Read the model definition and answer for the solid it produces. Units are mm, in the model's axes. A direction names the side the tool comes from. Round coordinates to 2 decimals unless told otherwise and drop trailing zeros. Write each loop counter-clockwise with the first axis right and the second up, starting at its lowest first coordinate (ties: lowest second). Pieces come first, ordered by that corner, then holes. Notation, with made-up numbers: (69, 80.5) - (75, 80.5) arc R33 cw to (75, 116.5) - close; hole circle Ø10 at (57, 1). An arc over 180 degrees is marked (long way). Use one line per item in the form item = value. Start each with the question number.
1) The part is cut by section C-C, the plane x = 60. Give the vertices of the cut face in (y, z).
2) The part is cut by section D-D, the plane y = -129.5. Give the vertices of the cut face in (x, z), plus the area to 3 significant figures.
3) Each of these flat-tipped pins is pushed along its axis until it touches: pin 1 (11 mm diameter, centred on x = 110, y = -73.5, fed in from -Z); pin 2 (6 mm diameter, centred on x = 11.5, z = 70, fed in from +Y); pin 3 (16 mm diameter, centred on x = 58, z = 13, fed in from -Y); pin 4 (2 mm diameter, centred on x = 89.5, y = -65, fed in from +Z). Where does it stop, or does it pass through?
4) The part is cut by section A-A, the plane y = -50.5. Give the vertices of the cut face in (x, z).
5) Consider line 1 along Y through (x, z) = (73, 228.5); line 2 along Z through (x, y) = (13, -100); line 3 along Y through (x, z) = (16, 213). Determine where each line is inside the solid, lowest interval first. Write a range as from..to.
6) For a pull along Z with two mould halves and no side action, classify faces 1 (the face through (113, -74, 170)), 2 (the face through (60, -48, 270)), 3 (the face through (25, -138, 10)) as released by +Z, released by -Z, zero draft, split by the parting line, or undercut.
7) For faces 4 (the face through (35, -23, 10)), 5 (the face through (30, -15, 233)), 6 (the face through (40, -20, 232)), determine the directions among +Z, -Z, +X, -X, +Y, -Y from which every point of the face is accessible in a straight line to the end or side of a thin tool.
8) The part is cut by section B-B, the plane z = 72.5. Give the vertices of the cut face in (x, y), plus the area to 3 significant figures.
from build123d import *

# Parameters (mm, degrees)
SKETCH_1_W          = 120
SKETCH_1_H          = 150
EXTRUDE_1_DEPTH     = 20
SKETCH_2_W          = 120
SKETCH_2_H          = 10
EXTRUDE_3_DEPTH     = 250
SKETCH_3_W          = 50
SKETCH_3_H          = 45
CUT_EXTRUDE_1_DEPTH = 316.277655409
SKETCH_4_W          = 70
SKETCH_4_H          = 25
CUT_EXTRUDE_2_DEPTH = 316.277655409
SKETCH_5_W          = 20
SKETCH_5_H          = 20
CUT_EXTRUDE_3_DEPTH = 3
CUT_EXTRUDE_START   = -100
CUT_EXTRUDE_6_DEPTH = 20
SKETCH_7_W          = 20
SKETCH_7_H          = 75
EXTRUDE_4_DEPTH     = 50
SKETCH_8_W          = 60
SKETCH_8_H          = 75
EXTRUDE_5_DEPTH     = 10


with BuildPart() as part:
    # Эскиз1 → Бобышка-Вытянуть1 (new body)
    with BuildSketch(Plane.XY):
        with Locations((60, -75)):
            Rectangle(SKETCH_1_W, SKETCH_1_H)
    extrude(amount=EXTRUDE_1_DEPTH)

    # Эскиз2 → Бобышка-Вытянуть3 (add)
    with BuildSketch(Plane.XY.offset(20)):
        with Locations((60, -75)):
            Rectangle(SKETCH_2_W, SKETCH_2_H)
    extrude(amount=EXTRUDE_3_DEPTH)

    # Эскиз3 → Вырез-Вытянуть1 (cut, through all)
    with BuildSketch(Plane.XY.offset(20)):
        with Locations((60, -22.5)):
            Rectangle(SKETCH_3_W, SKETCH_3_H)
    extrude(amount=-CUT_EXTRUDE_1_DEPTH, mode=Mode.SUBTRACT)

    # Эскиз4 → Вырез-Вытянуть2 (cut, through all)
    with BuildSketch(Plane.XY.offset(20)):
        with Locations((60, -137.5)):
            Rectangle(SKETCH_4_W, SKETCH_4_H)
    extrude(amount=-CUT_EXTRUDE_2_DEPTH, mode=Mode.SUBTRACT)

    # Эскиз5 → Вырез-Вытянуть3 (cut)
    with BuildSketch(Plane(origin=(0, -70, 0), x_dir=(1, 0, 0), z_dir=(0, 1, 0))):
        with Locations((10, -72.859885292)):
            Rectangle(SKETCH_5_W, SKETCH_5_H)
    extrude(amount=-CUT_EXTRUDE_3_DEPTH, mode=Mode.SUBTRACT)

    # Эскиз6 → Вырез-Вытянуть6 (cut)
    with BuildSketch(Plane.XY.offset(270).offset(CUT_EXTRUDE_START)):
        Polygon((120, -80), (102.679491924, -70), (120, -70), align=None)
    extrude(amount=-CUT_EXTRUDE_6_DEPTH, mode=Mode.SUBTRACT)

    # Эскиз7 → Бобышка-Вытянуть4 (add)
    with BuildSketch(Plane(origin=(0, -70, 0), x_dir=(1, 0, 0), z_dir=(0, 1, 0))):
        with Locations((60, -232.5)):
            Rectangle(SKETCH_7_W, SKETCH_7_H)
    extrude(amount=EXTRUDE_4_DEPTH)

    # Эскиз8 → Бобышка-Вытянуть5 (add)
    with BuildSketch(Plane(origin=(0, -20, 0), x_dir=(1, 0, 0), z_dir=(0, 1, 0))):
        with Locations((60, -232.5)):
            Rectangle(SKETCH_8_W, SKETCH_8_H)
    extrude(amount=EXTRUDE_5_DEPTH)


solid = part.part
Geometry results:
q1.outline = (-125, 0) - (-45, 0) - (-45, 20) - (-70, 20) - (-70, 195) - (-10, 195) - (-10, 270) - (-80, 270) - (-80, 20) - (-125, 20) - close
q2.outline = (0, 0) - (25, 0) - (25, 20) - (0, 20) - close; (95, 0) - (120, 0) - (120, 20) - (95, 20) - close
q2.area = 1,000 mm2
q3.pin_1 = 0
q3.pin_2 = -73
q3.pin_3 = -125
q3.pin_4 = 20
q4.outline = (0, 0) - (120, 0) - (120, 20) - (0, 20) - close; (50, 195) - (70, 195) - (70, 270) - (50, 270) - close
q5.line_1 = -80..-70, -20..-10
q5.line_2 = 0..20
q5.line_3 = -80..-70
q6.face_1 = undercut
q6.face_2 = released by +Z
q6.face_3 = zero draft
q7.face_4 = -Z, +Y
q7.face_5 = +Z, -X, +Y
q7.face_6 = +Z, -X
q8.outline = (0, -80) - (120, -80) - (120, -70) - (20, -70) - (20, -73) - (0, -73) - close
q8.area = 1,140 mm2
